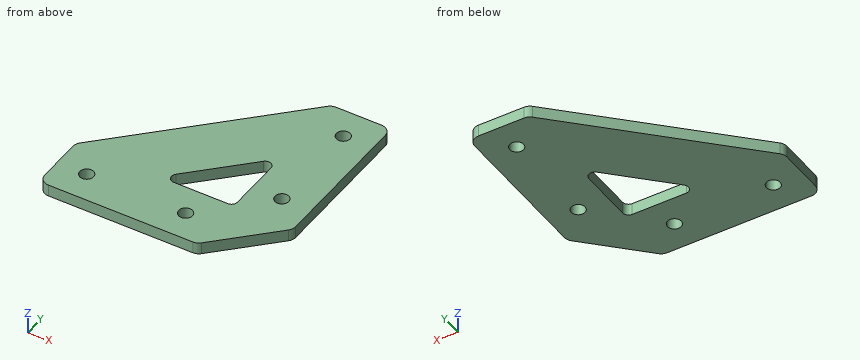
```python
from build123d import *

# Parameters (mm, degrees)
SKETCH_R    = 3.5
PAD_DEPTH   = 6
FILLET_R    = 5
FILLET001_R = 3


with BuildPart() as part:
    # Sketch → Pad (new body)
    with BuildSketch(Plane.XY):
        Polygon((-30, 0), (-110, 0), (-110, 30), (-30, 110), (0, 110), (0, 30), align=None)
        with Locations((-95, 15)):
            Circle(SKETCH_R, mode=Mode.SUBTRACT)
        with Locations((-45, 15)):
            Circle(SKETCH_R, mode=Mode.SUBTRACT)
        with Locations((-15, 45)):
            Circle(SKETCH_R, mode=Mode.SUBTRACT)
        with Locations((-15, 95)):
            Circle(SKETCH_R, mode=Mode.SUBTRACT)
        Polygon((-30, 67.573593), (-67.573593, 30), (-30, 30), align=None, mode=Mode.SUBTRACT)
    extrude(amount=PAD_DEPTH)

    # Fillet
    fillet_edges = [part.edges().sort_by_distance(p)[0] for p in [
        (-110, 0, 3),
        (-110, 30, 3),
        (-30, 110, 3),
        (0, 110, 3),
        (0, 30, 3),
        (-30, 0, 3),
    ]]
    fillet(fillet_edges, radius=FILLET_R)

    # Fillet001
    fillet001_edges = [part.edges().sort_by_distance(p)[0] for p in [
        (-67.573593, 30, 3),
        (-30, 67.573593, 3),
        (-30, 30, 3),
    ]]
    fillet(fillet001_edges, radius=FILLET001_R)


solid = part.part
```
The listing builds one solid part. Answer for the finished solid, in the listing's coordinates (mm). Round coordinates to 2 decimals unless told otherwise and drop trailing zeros. Order: outer loops, then holes, each group sorted by start corner. A loop starts at its lowest first (then second) coordinate and runs counter-clockwise, first axis right, second up. Notation, with made-up numbers: (-17, 68.5) -> (-8, 68.5) arc R23 cw to (-8, 105.5) -> close; hole circle Ø7 at (63, 7.25). An arc over 180 degrees is marked (long way). Answer as CSV lines item,"result". Start each with the question number.
(1) Find the intervals of material crossed by probe 1 along X at (y, z) = (13, 5.55); probe 2 along Y at (x, z) = (-44, 1.75); probe 3 along X at (y, z) = (60.5, 1.9), in increasing order. Write a range as from..to.
(2) The part is cut by section D-D (y = 95). Determine the outline of the cut face in (x, z), then the cut area to 3 significant figures.
(3) Flat-ended cylindrical pins translate along their axes: pin 1 Ø1 at (y, z) = (73, 1.5) entering from -X; pin 2 Ø2 at (y, z) = (61.5, 1) entering from -X; pin 3 Ø1 at (y, z) = (89, 5) entering from -X. Find the tip coordinate at first contact, or state that the pin passes through.
(4) The part is cut by section B-B (y = 15). Determine the outline of the cut face in (x, z).
(5) The part is cut by section C-C (z = 4.25). Determine the outline of the cut face in (x, y), then the cut area to 3 significant figures.
(6) The part is cut by section A-A (x = -15). Determine the outline of the cut face in (y, z), then the cut area to 3 significant figures.
Evaluation:
1,probe 1,"-110..-97.87, -92.13..-47.87, -42.13..-17"
1,probe 2,"0..11.65, 18.35..30, 53.57..96"
1,probe 3,"-79.5..-37.07, -30..0"
2,outline,"(-45, 0) -> (-18.5, 0) -> (-18.5, 6) -> (-45, 6) -> close; (-11.5, 0) -> (0, 0) -> (0, 6) -> (-11.5, 6) -> close"
2,area,"228 mm²"
3,pin 1,"x = -67.5"
3,pin 2,"x = -79.5"
3,pin 3,"x = -51.5"
4,outline,"(-110, 0) -> (-98.5, 0) -> (-98.5, 6) -> (-110, 6) -> close; (-91.5, 0) -> (-48.5, 0) -> (-48.5, 6) -> (-91.5, 6) -> close; (-41.5, 0) -> (-15, 0) -> (-15, 6) -> (-41.5, 6) -> close"
5,outline,"(-110, 5) arc R5 ccw to (-105, 0) -> (-32.07, 0) arc R5 ccw to (-28.54, 1.46) -> (-1.46, 28.54) arc R5 ccw to (0, 32.07) -> (0, 105) arc R5 ccw to (-5, 110) -> (-27.93, 110) arc R5 ccw to (-31.46, 108.54) -> (-108.54, 31.46) arc R5 ccw to (-110, 27.93) -> close; hole circle Ø7 at (-95, 15); hole (-62.45, 35.12) arc R3 ccw to (-60.33, 30) -> (-33, 30) arc R3 ccw to (-30, 33) -> (-30, 60.33) arc R3 ccw to (-35.12, 62.45) -> close; hole circle Ø7 at (-45, 15); hole circle Ø7 at (-15, 45); hole circle Ø7 at (-15, 95)"
5,area,"7,600 mm²"
6,outline,"(15, 0) -> (41.5, 0) -> (41.5, 6) -> (15, 6) -> close; (48.5, 0) -> (91.5, 0) -> (91.5, 6) -> (48.5, 6) -> close; (98.5, 0) -> (110, 0) -> (110, 6) -> (98.5, 6) -> close"
6,area,"486 mm²"
